Source: CAD feature listing. Evaluate the final solid. Frame: model axes, mm. A direction names the side the tool comes from. Round coordinates to 2 decimals unless told otherwise and drop trailing zeros. Write each loop counter-clockwise with the first axis right and the second up, starting at its lowest first coordinate (ties: lowest second). Pieces come first, ordered by that corner, then holes. Notation, with made-up numbers: M -30.75,50 L 7.25,50 A11 cw 7.25,61 Z; hole C 73.5,65 d10. An arc over 180 degrees is marked long. Put each result on its own line as item: value. Start each with the question number.
Solid Edge part; units mm, degrees
sketch "Sketch1" plane through (0, 0, 0) normal (0, 0, 1) x (1, 0, 0)
  line L0 (51.1, -41.5) -> (51.1, 41.5)
  line L1 (51.1, 41.5) -> (-51.1, 41.5)
  line L2 (-51.1, 41.5) -> (-51.1, -41.5)
  line L3 (-51.1, -41.5) -> (51.1, -41.5)
extrude "Protrusion1" add sketch "Sketch1" along normal blind 14.54
sketch "Sketch2" plane through (0, 0, 14.54) normal (0, 0, 1) x (1, 0, 0)
  line L0 (49.1, -39.5) -> (49.1, 39.5)
  line L1 (49.1, 39.5) -> (-49.1, 39.5)
  line L2 (-49.1, 39.5) -> (-49.1, -39.5)
  line L3 (-49.1, -39.5) -> (49.1, -39.5)
extrude "ProtrusiónExtruida_2" add sketch "Sketch2" along normal blind 2
sketch "Sketch3" plane through (0, 0, 16.54) normal (0, 0, 1) x (1, 0, 0)
  line L0 (48.1, -38.5) -> (48.1, 38.5)
  line L1 (48.1, 38.5) -> (-48.1, 38.5)
  line L2 (-48.1, 38.5) -> (-48.1, -38.5)
  line L3 (-48.1, -38.5) -> (48.1, -38.5)
extrude "VaciadoExtruido_1" cut sketch "Sketch3" against normal blind 8
sketch "Sketch4" plane through (0, 0, 8.54) normal (0, 0, 1) x (1, 0, 0)
  circle A0 centre (42.5, 25) radius 1.7
  circle A1 centre (42.5, 25) radius 1.2
  circle A2 centre (-42.5, -25) radius 1.7
  circle A3 centre (-42.5, -25) radius 1.2
extrude "ProtrusiónExtruida_5" add sketch "Sketch4" along normal blind 6
sketch "Sketch5" plane through (0, 0, 8.54) normal (0, 0, 1) x (1, 0, 0)
  line L0 (-6, -35.5) -> (-6, -17.5)
  line L1 (-6, -17.5) -> (-4, -17.5)
  line L2 (-4, -17.5) -> (-4, -35.5)
  line L3 (-4, -35.5) -> (-6, -35.5)
  line L4 (6, -35.5) -> (6, -17.5)
  line L5 (6, -17.5) -> (4, -17.5)
  line L6 (4, -17.5) -> (4, -35.5)
  line L7 (4, -35.5) -> (6, -35.5)
extrude "VaciadoExtruido_3" cut sketch "Sketch5" against normal blind 60
sketch "Sketch6" plane through (0, 0, 8.54) normal (0, 0, 1) x (1, 0, 0)
  circle A0 centre (0.5, -20.6929) radius 0.5
extrude "VaciadoExtruido_4" cut sketch "Sketch6" against normal blind 60
sketch "Sketch7" plane through (0, 0, 8.54) normal (0, 0, 1) x (1, 0, 0)
  line L0 (47.1689, 15) -> (17.1689, 15)
  line L1 (17.1689, 15) -> (17.1689, 11)
  line L2 (17.1689, 11) -> (47.1689, 11)
  line L3 (47.1689, 11) -> (47.1689, 15)
  line L4 (-47.1689, 15) -> (-17.1689, 15)
  line L5 (-17.1689, 15) -> (-17.1689, 11)
  line L6 (-17.1689, 11) -> (-47.1689, 11)
  line L7 (-47.1689, 11) -> (-47.1689, 15)
extrude "VaciadoExtruido_5" cut sketch "Sketch7" against normal blind 61.0922
sketch "Sketch8" plane through (51.1, 0, 7.27) normal (1, 0, 0) x (0, 1, 0)
  line L0 (5, 9.27) -> (5, -7.27)
  line L1 (5, -7.27) -> (-5, -7.27)
  line L2 (-5, -7.27) -> (-5, 9.27)
  line L3 (-5, 9.27) -> (5, 9.27)
extrude "VaciadoExtruido_7" cut sketch "Sketch8" against normal blind 3.3
sketch "Sketch9" plane through (0, 0, 8.54) normal (0, 0, 1) x (1, 0, 0)
  line L0 (47.7, 5.5178) -> (47.7, -5.6822)
  line L1 (47.7, -5.6822) -> (46.2, -5.6822)
  line L2 (46.2, -5.6822) -> (46.2, 5.5178)
  line L3 (46.2, 5.5178) -> (47.7, 5.5178)
extrude "ProtrusiónExtruida_6" add sketch "Sketch9" along normal blind 16.54
sketch "Sketch10" plane through (46.95, -5.6822, 16.81) normal (0, -1, 0) x (0, 0, -1)
  line L0 (-8.27, 0.75) -> (-5.8337, 3.6691)
  line L1 (-5.8337, 3.6691) -> (-5.8337, 0.75)
  line L2 (-5.8337, 0.75) -> (-8.27, 0.75)
extrude "ProtrusiónExtruida_8" add sketch "Sketch10" against normal blind 11.2
sketch "Sketch11" plane through (46.2, -0.0822, 16.81) normal (-1, 0, 0) x (0, -1, 0)
  line L0 (5.6, -0.73) -> (5.6, 8.27)
  line L1 (5.6, 8.27) -> (4.1, 8.27)
  line L2 (4.1, 8.27) -> (4.1, -0.73)
  line L3 (4.1, -0.73) -> (5.6, -0.73)
  line L4 (-4.1, 8.27) -> (-4.1, -0.73)
  line L5 (-4.1, -0.73) -> (-5.6, -0.73)
  line L6 (-5.6, -0.73) -> (-5.6, 8.27)
  line L7 (-5.6, 8.27) -> (-4.1, 8.27)
extrude "Cutout1" cut sketch "Sketch11" against normal blind 34.3591
sketch "Sketch12" plane through (0, -41.5, 7.27) normal (0, -1, 0) x (1, 0, 0)
  line L0 (-5, -7.27) -> (-5, -2.27)
  line L1 (-5, -2.27) -> (5, -2.27)
  line L2 (5, -2.27) -> (5, -7.27)
  line L3 (5, -7.27) -> (-5, -7.27)
extrude "VaciadoExtruido_18" cut sketch "Sketch12" against normal blind 10000
sketch "Sketch13" plane through (51.1, 23.25, 7.27) normal (1, 0, 0) x (0, 1, 0)
  line L0 (-5.5, -2.27) -> (-5.5, -7.27)
  line L1 (-5.5, -7.27) -> (-41, -7.27)
  line L2 (-41, -7.27) -> (-41, -2.27)
  line L3 (-41, -2.27) -> (-5.5, -2.27)
extrude "Cutout2" cut sketch "Sketch13" against normal blind 100000
sketch "Sketch14" plane through (-48.1, 0, 12.54) normal (1, 0, 0) x (0, 1, 0)
  line L0 (5, -12.54) -> (5, 4)
  line L1 (5, 4) -> (-5, 4)
  line L2 (-5, 4) -> (-5, -12.54)
  line L3 (-5, -12.54) -> (5, -12.54)
extrude "Cutout3" cut sketch "Sketch14" against normal blind 3.3
sketch "Sketch15" plane through (0, 0, 8.54) normal (0, 0, 1) x (0, 1, 0)
  line L0 (5.6, 46.6) -> (-5.6, 46.6)
  line L1 (-5.6, 46.6) -> (-5.6, 48.1)
  line L2 (-5.6, 48.1) -> (5.6, 48.1)
  line L3 (5.6, 48.1) -> (5.6, 46.6)
extrude "ProtrusiónExtruida_9" add sketch "Sketch15" along normal blind 16.54
sketch "Sketch16" plane through (-47.35, -5.6, 16.81) normal (0, -1, 0) x (0, 0, 1)
  line L0 (8.27, 0.75) -> (6.3463, 2.4083)
  line L1 (6.3463, 2.4083) -> (6.3463, 0.75)
  line L2 (6.3463, 0.75) -> (8.27, 0.75)
extrude "Protrusion2" add sketch "Sketch16" against normal up to vertex (11.2 mm away)
sketch "Sketch17" plane through (-46.6, 0, 16.81) normal (1, 0, 0) x (0, 1, 0)
  line L0 (-4.1, 8.27) -> (-4.1, -0.73)
  line L1 (-4.1, -0.73) -> (-5.6, -0.73)
  line L2 (-5.6, -0.73) -> (-5.6, 8.27)
  line L3 (-5.6, 8.27) -> (-4.1, 8.27)
  line L4 (4.1, 8.27) -> (4.1, -0.73)
  line L5 (4.1, -0.73) -> (5.6, -0.73)
  line L6 (5.6, -0.73) -> (5.6, 8.27)
  line L7 (5.6, 8.27) -> (4.1, 8.27)
extrude "Cutout4" cut sketch "Sketch17" against normal blind 20988
(1) Pull-direction query (Z, two-part tool) for faces 1 (the flat face through (47.7, 0, 15)), 2 (the flat face through (46.2, 0, 17)), 3 (the flat face through (28, -29, 0)); classes: +Z half, -Z half, draft (parallel to the pull), parting line (faces both ways), or undercut.
(2) Section query A-A (z = 13.25). Return loops of the section in (x, y).
(3) Ray query, line 1 along Y through (x, z) = (-42.5, 9.9); line 2 along Y through (x, z) = (42.5, 11.75); line 3 along Y through (x, z) = (0.5, 6.3). Return the intervals inside material, ascending.
(4) Access query for faces 4 (the flat face through (-50, -5, 11)), 5 (the flat face through (-4, -26, 7)), 6 (the flat face through (48.1, -22, 13)), 7 (the flat face through (28, 17.75, 3)), 8 (the flat face through (49, 5, 11)). Directions: +Z, -Z, +X, -X, +Y, -Y. A direction counts if a zero-diameter tool reaches every point of the face in a straight line with its end or side. Return the directions, or none.
(5) Section query C-C (x = 36). Return loops of the section in (y, z).
(6) Section query B-B (y = -25). Return loops of the section in (x, z), and give its area (3 significant figures).
(7) Contact query for flat-ended pins moving along their axis: P1, Ø0.8, axis at x = 49, y = -5.5, coming from the +Z side; P2, Ø1.2, axis at x = -42.5, y = -25.5, coming from the +Z side; P3, Ø2.5, axis at x = 42.5, y = 24.5, coming from the +Z side. Output: stop coordinate, or through.
(8) Section query D-D (z = 18.75). Return loops of the section in (x, y), and give its area (3 significant figures).
Entries:
1. face 1: undercut
1. face 2: draft
1. face 3: -Z half
2. outline: M -51.1,-41.5 L 51.1,-41.5 L 51.1,-5 L 48.1,-5 L 48.1,-38.5 L -48.1,-38.5 L -48.1,-5.6 L -46.6,-5.6 L -46.6,5.6 L -48.1,5.6 L -48.1,38.5 L 48.1,38.5 L 48.1,5 L 51.1,5 L 51.1,41.5 L -51.1,41.5 L -51.1,5 L -48.1,5 L -48.1,-5 L -51.1,-5 Z; C -42.5,-25 d3.4; C 42.5,25 d3.4; M 46.2,-5.68 L 47.7,-5.68 L 47.7,5.52 L 46.2,5.52 Z; hole C -42.5,-25 d2.4; hole C 42.5,25 d2.4
3. line 1: -41.5 to -38.5, -26.7 to -26.2, -23.8 to -23.3, 38.5 to 41.5
3. line 2: -41.5 to -38.5, 23.3 to 23.8, 26.2 to 26.7, 38.5 to 41.5
3. line 3: -41.5 to -21.19, -20.19 to 41.5
4. face 4: +Z, -Z, -X
4. face 5: +Z, -Z
4. face 6: +Z
4. face 7: -Z, +X, -X
4. face 8: +Z, -Z, +X
5. outline: M -41.5,0 L -17.75,0 L -17.75,5 L 11,5 L 11,8.54 L -38.5,8.54 L -38.5,16.54 L -39.5,16.54 L -39.5,14.54 L -41.5,14.54 Z; M 15,5 L 17.75,5 L 17.75,0 L 41.5,0 L 41.5,14.54 L 39.5,14.54 L 39.5,16.54 L 38.5,16.54 L 38.5,8.54 L 15,8.54 Z
6. outline: M -51.1,0 L -6,0 L -6,8.54 L -40.8,8.54 L -40.8,14.54 L -41.3,14.54 L -41.3,8.54 L -43.7,8.54 L -43.7,14.54 L -44.2,14.54 L -44.2,8.54 L -48.1,8.54 L -48.1,16.54 L -49.1,16.54 L -49.1,14.54 L -51.1,14.54 Z; M -4,5 L 4,5 L 4,8.54 L -4,8.54 Z; M 6,0 L 51.1,0 L 51.1,14.54 L 49.1,14.54 L 49.1,16.54 L 48.1,16.54 L 48.1,8.54 L 6,8.54 Z
6. area: 845 mm2
7. P1: z = 16.54
7. P2: z = 8.54
7. P3: z = 14.54
8. outline: M -48.1,-4.1 L -46.6,-4.1 L -46.6,4.1 L -48.1,4.1 Z; M 46.2,-4.18 L 47.7,-4.18 L 47.7,4.02 L 46.2,4.02 Z
8. area: 24.6 mm2
